The drawing under review shows one solid part. Ordinate dimensions are in mm from its lowest x, y, z. A direction names the side the tool comes from. Round coordinates to 2 decimals unless told otherwise and drop trailing zeros. Write each loop counter-clockwise with the first axis right and the second up, starting at its lowest first coordinate (ties: lowest second). Pieces come first, ordered by that corner, then holes. Notation, with made-up numbers: (-37.5, 30) -> (-29.5, 30) arc R13 ccw to (-29.5, 47) -> close; hole circle Ø4 at (24, -6.5). An arc over 180 degrees is marked (long way). Answer in a Markdown table with one row per item.
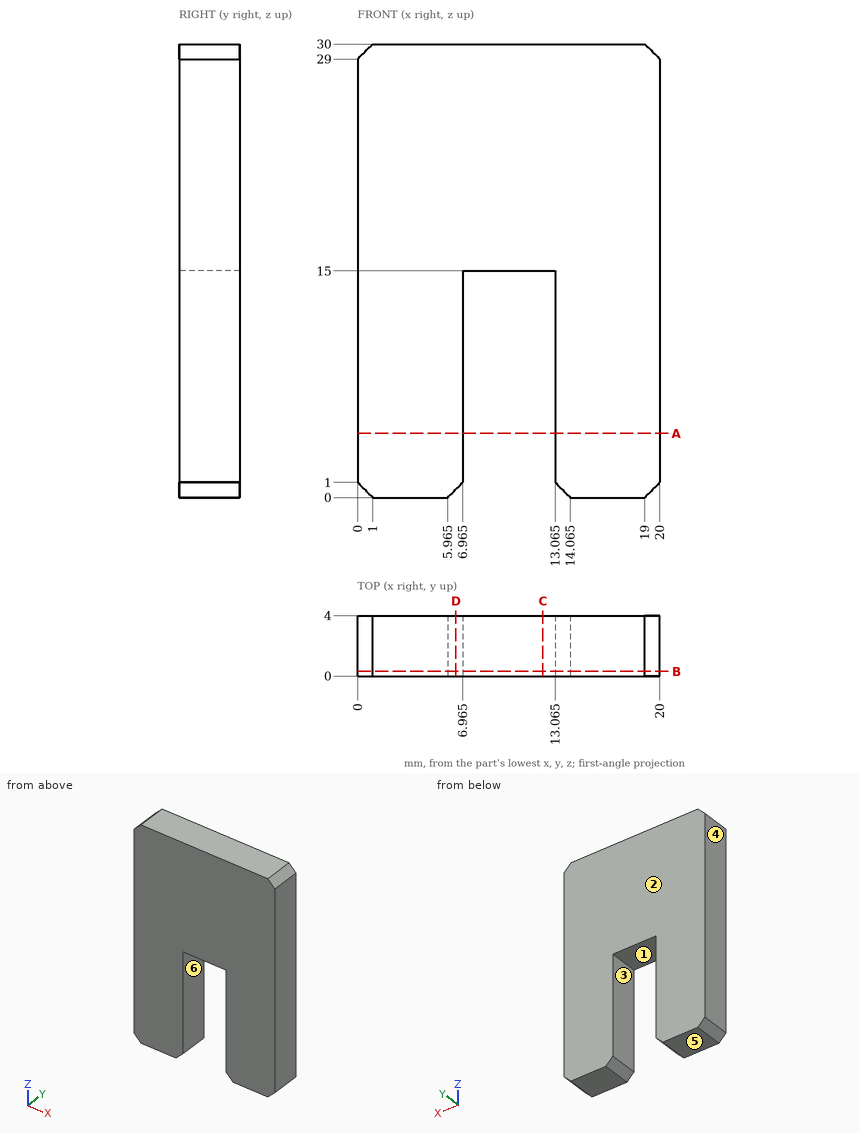
1) For the marked faces 1 and 2, list the 3-axis set-ups (+Z, -Z, +X, -X, +Y, -Y) from which the entire face can be reached by the end or side of a thin tool; tool diameter is ignored.
Solved:
| item | result |
|---|---|
| face 1 | -Z, +Y, -Y |
| face 2 | +Z, -Z, +X, -X, +Y |
2) For line 1 (X direction, y = 1.7, z = 14) (1 decimal); line 2 (Z direction, x = 10.5, y = 2.8), list the stretches that pass through material, from the lowest coordinate up. Write a range as [from, to].
Solved:
| item | result |
|---|---|
| line 1 | [0, 7], [13.1, 20] |
| line 2 | [15, 30] |
3) Consider section D-D on x = 6.5. State the section outline as (y, z) points (1 decimal).
Solved:
| item | result |
|---|---|
| outline | (0, 0.5) -> (4, 0.5) -> (4, 30) -> (0, 30) -> close |
4) Consider section B-B on y = 0.3. State the section outline as (x, z) points (1 decimal).
Solved:
| item | result |
|---|---|
| outline | (0, 1) -> (1, 0) -> (6, 0) -> (7, 1) -> (7, 15) -> (13.1, 15) -> (13.1, 1) -> (14.1, 0) -> (19, 0) -> (20, 1) -> (20, 29) -> (19, 30) -> (1, 30) -> (0, 29) -> close |
5) Mouldability with a two-part tool opening along X and no side actions: class the marked faces 3, 4, 5 and 6 as pulls with the +X half, pulls with the -X half, needs draft (parallel to the pull), parting line crosses it, or undercut.
Solved:
| item | result |
|---|---|
| face 3 | undercut |
| face 4 | pulls with the -X half |
| face 5 | needs draft |
| face 6 | undercut |
6) Consider section C-C on x = 12.25. State the section outline as (y, z) points, then the cut area to 3 significant figures.
Solved:
| item | result |
|---|---|
| outline | (0, 15) -> (4, 15) -> (4, 30) -> (0, 30) -> close |
| area | 60.0 mm² |
7) Clearance check with flat-ended pins moving along their axes: pin 1 Ø1.2 at (x, y) = (10.5, 1.5) entering from -Z; pin 2 Ø1 at (x, z) = (8, 15.5) entering from -Y. State where each tip first meets the part, or that it passes through.
Solved:
| item | result |
|---|---|
| pin 1 | z = 15 |
| pin 2 | y = 0 |
8) Consider section A-A on z = 4.25. State the section outline as (x, y) points (1 decimal).
Solved:
| item | result |
|---|---|
| outline | (0, 0) -> (7, 0) -> (7, 4) -> (0, 4) -> close; (13.1, 0) -> (20, 0) -> (20, 4) -> (13.1, 4) -> close |
